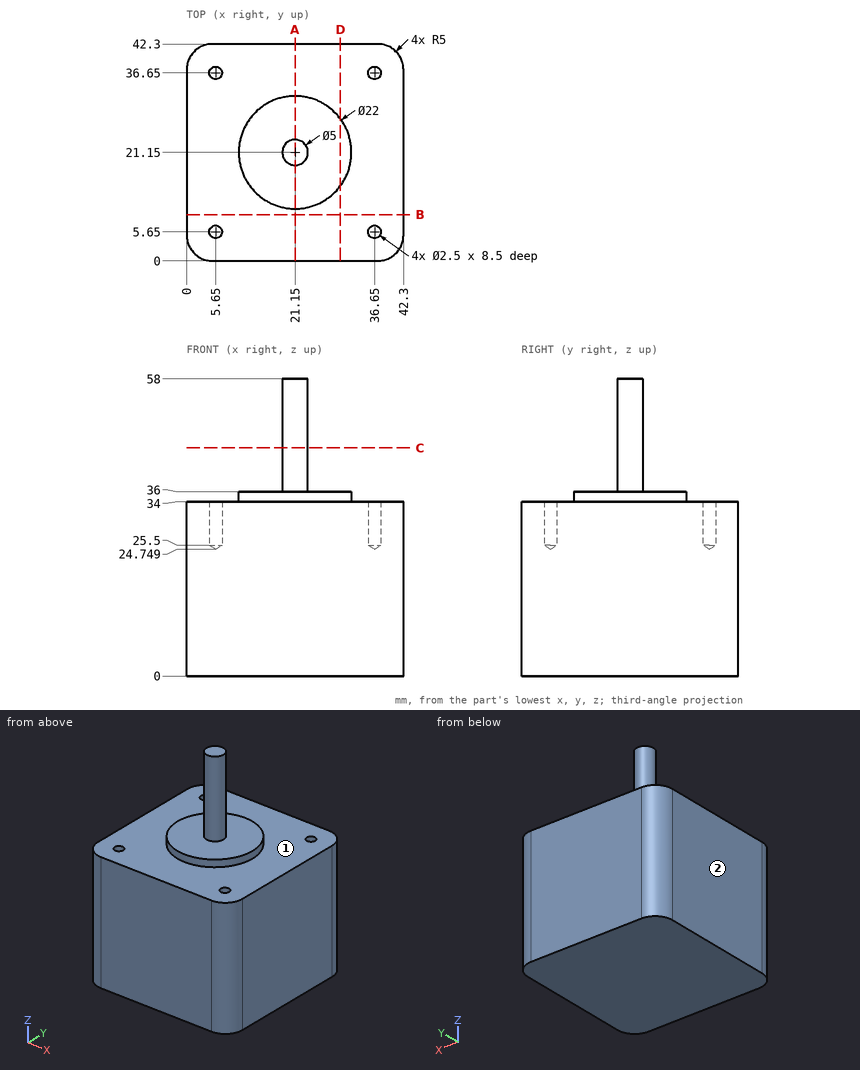
Geometry: see drawing. Coordinates: mm, zero at the bounding-box minimum. A direction names the side the tool comes from. Coordinates: 2 decimals unless noted, no trailing zeros. Loops run counter-clockwise (first coordinate to the right, second up) from the corner with the lowest first, then second, coordinate; pieces in that order, holes last. Notation, with made-up numbers: M -26,46 L 9,46 A23 cw 9,71 Z; hole C -0.75,-1.5 d7. An arc over 180 degrees is marked long. Put each result on its own line as item: value. Start each with the question number.
1) Contact query for flat-ended pins moving along their axis: pin 1 Ø8 at (x, y) = (9, 15) entering from +Z; pin 2 Ø4 at (x, y) = (36.65, 5.65) entering from +Z; pin 3 Ø2 at (x, y) = (5.65, 36.65) entering from +Z; pin 4 Ø5 at (y, z) = (15.5, 49.5) entering from +X. Output: stop coordinate, or through.
2) Cut plane B-B on y = 9. Return the cut outline in (x, z).
3) Cut plane A-A on x = 21.15. Return the cut outline in (y, z).
4) Reachability of the marked faces 1 and 2 from +Z, -Z, +X, -X, +Y, -Y: full face, straight path, thin tool, end or side. Return the list, or none.
5) Cut plane D-D on x = 30. Return the cut outline in (y, z), then the cut area to 3 significant figures.
6) Cut plane C-C on z = 44.5. Return the cut outline in (x, y).
7) Ray query, L1, parallel to Y at x = 36.65, z = 29; L2, parallel to Z at x = 13, y = 37. Return the intervals inside material, ascending. Write a range as from..to.
The answers:
1. pin 1: stops at z = 36
1. pin 2: stops at z = 34
1. pin 3: stops at z = 25.35
1. pin 4: passes through
2. outline: M 0,0 L 42.3,0 L 42.3,34 L 0,34 Z
3. outline: M 0,0 L 42.3,0 L 42.3,34 L 32.15,34 L 32.15,36 L 23.65,36 L 23.65,58 L 18.65,58 L 18.65,36 L 10.15,36 L 10.15,34 L 0,34 Z
4. face 1: +Z
4. face 2: +Z, -Z, -X, +Y, -Y
5. outline: M 0,0 L 42.3,0 L 42.3,34 L 27.68,34 L 27.68,36 L 14.62,36 L 14.62,34 L 0,34 Z
5. area: 1,460 mm²
6. outline: C 21.15,21.15 d5
7. L1: y = 0..4.4, 6.9..35.4, 37.9..42.3
7. L2: z = 0..34
